The model under review builds one solid part; all positions refer to its coordinate system, in mm. A direction names the side the tool comes from. Round coordinates to 2 decimals unless told otherwise and drop trailing zeros. Order: outer loops, then holes, each group sorted by start corner. A loop starts at its lowest first (then second) coordinate and runs counter-clockwise, first axis right, second up. Notation, with made-up numbers: (43, 39.5) -> (95, 39.5) arc R7 ccw to (95, 45.5) -> close; hole circle Ø10 at (26.25, -31.5). An arc over 180 degrees is marked (long way). Use a Markdown table: item, result. Add a question column.
```python
from build123d import *

# Parameters (mm, degrees)
CROQUIS1_W              = 50
CROQUIS1_H              = 44
SALIENTE_EXTRUIR1_DEPTH = 10
CROQUIS2_W              = 58
CROQUIS2_H              = 22.5
CORTAR_EXTRUIR2_DEPTH   = 2
CROQUIS3_W              = 25
CROQUIS3_H              = 22.5
CORTAR_EXTRUIR3_DEPTH   = 4
CROQUIS4_R              = 1.1
CORTAR_EXTRUIR4_DEPTH   = 5
CROQUIS5_R              = 1.1
CORTAR_EXTRUIR5_DEPTH   = 5
REDONDEO1_R             = 2
REDONDEO2_R             = 1


with BuildPart() as part:
    # Croquis1 → Saliente-Extruir1 (new body)
    with BuildSketch(Plane(origin=(0, 0, 0), x_dir=(1, 0, 0), z_dir=(0, 1, 0))):
        Rectangle(CROQUIS1_W, CROQUIS1_H)
    extrude(amount=SALIENTE_EXTRUIR1_DEPTH)

    # Croquis2 → Cortar-Extruir2 (cut)
    with BuildSketch(Plane(origin=(0, 10, 0), x_dir=(1, 0, 0), z_dir=(0, 1, 0))):
        Rectangle(CROQUIS2_W, CROQUIS2_H)
    extrude(amount=-CORTAR_EXTRUIR2_DEPTH, mode=Mode.SUBTRACT)

    # Croquis3 → Cortar-Extruir3 (cut)
    with BuildSketch(Plane(origin=(0, 8, 0), x_dir=(1, 0, 0), z_dir=(0, 1, 0))):
        Rectangle(CROQUIS3_W, CROQUIS3_H)
    extrude(amount=-CORTAR_EXTRUIR3_DEPTH, mode=Mode.SUBTRACT)

    # Croquis4 → Cortar-Extruir4 (cut)
    with BuildSketch(Plane(origin=(0, 8, 0), x_dir=(1, 0, 0), z_dir=(0, 1, 0))):
        with Locations(Location((-22.5, 8, 0), (0, 0, 270))):
            Circle(CROQUIS4_R)
        with Locations(Location((-22.5, -8, 0), (0, 0, 270))):
            Circle(CROQUIS4_R)
        with Locations(Location((22.5, 8, 0), (0, 0, 270))):
            Circle(CROQUIS4_R)
        with Locations(Location((22.5, -8, 0), (0, 0, 270))):
            Circle(CROQUIS4_R)
    extrude(amount=-CORTAR_EXTRUIR4_DEPTH, mode=Mode.SUBTRACT)

    # Croquis5 → Cortar-Extruir5 (cut)
    with BuildSketch(Plane(origin=(0, 10, 0), x_dir=(1, 0, 0), z_dir=(0, 1, 0))):
        with Locations(Location((0, 16.625, 0), (0, 0, 270))):
            Circle(CROQUIS5_R)
        with Locations(Location((0, -16.625, 0), (0, 0, 270))):
            Circle(CROQUIS5_R)
    extrude(amount=-CORTAR_EXTRUIR5_DEPTH, mode=Mode.SUBTRACT)

    # Redondeo1
    redondeo1_edges = [part.edges().sort_by_distance(p)[0] for p in [
        (-25, 5, -22),
        (25, 5, -22),
        (25, 5, 22),
        (-25, 5, 22),
    ]]
    fillet(redondeo1_edges, radius=REDONDEO1_R)

    # Redondeo2
    redondeo2_edges = [part.edges().sort_by_distance(p)[0] for p in [
        (0, 10, 11.25),
        (0, 10, -11.25),
    ]]
    fillet(redondeo2_edges, radius=REDONDEO2_R)


solid = part.part
```
Q1. Add section B-B (z = 8). Write out the cut boundary in (x, y).
Q2. Insertion check: pin 1 (1.8 mm diameter, centred on x = 22.5, z = -7.5, fed in from +Y); pin 2 (7 mm diameter, centred on x = 4, z = -3, fed in from +Y). Each pin has a flat end and moves straight along its axis. Give the tip position at first contact, or say it passes through.
Q3. Mouldability with a two-part tool opening along X and no side actions: class faces 1 (the cylindrical face through (21.426, 5.535, 7.762)), 2 (the flat face through (0, 7, -11.25)), 3 (the flat face through (-19, 8, 0)), 4 (the cylindrical face through (24.4, 5.07, 21.43)) as pulls with the +X half, pulls with the -X half, needs draft (parallel to the pull), parting line crosses it, or undercut.
Q4. Machinability: for faces 5 (the flat face through (23, 3, 8)), 6 (the flat face through (0, 10, -18)), which of the approach directions +Z, -Z, +X, -X, +Y, -Y give a long, thin tool a straight path to every point of the face, cutting with its end or side? Answer none if there is none.
Q5. Wall thickness on line 1 (X direction, y = 5.7, z = 8); line 2 (Z direction, x = 5, y = 8.25); line 3 (Y direction, x = 9.5, z = 9): over which ranges is each line inside the solid? List them lowest first. Write a range as [from, to].
Q6. Add section D-D (x = -20). Write out the cut boundary in (y, z).
Q7. Add section A-A (y = 6). Write out the cut boundary in (x, z) (3 decimals).
Q8. Add section C-C (x = -2). Write out the cut boundary in (y, z).
Report:
| question | item | result |
|---|---|---|
| 1 | outline | (-25, 0) -> (25, 0) -> (25, 8) -> (23.6, 8) -> (23.6, 3) -> (21.4, 3) -> (21.4, 8) -> (12.5, 8) -> (12.5, 4) -> (-12.5, 4) -> (-12.5, 8) -> (-21.4, 8) -> (-21.4, 3) -> (-23.6, 3) -> (-23.6, 8) -> (-25, 8) -> close |
| 2 | pin 1 | stops at y = 8 |
| 2 | pin 2 | stops at y = 4 |
| 3 | face 1 | undercut |
| 3 | face 2 | undercut |
| 3 | face 3 | needs draft |
| 3 | face 4 | pulls with the +X half |
| 4 | face 5 | +Y |
| 4 | face 6 | +Z, -Z, +X, -X, +Y |
| 5 | line 1 | x = [-25, -23.6], [-21.4, -12.5], [12.5, 21.4], [23.6, 25] |
| 5 | line 2 | z = [-22, -11.25], [11.25, 22] |
| 5 | line 3 | y = [0, 4] |
| 6 | outline | (0, -22) -> (10, -22) -> (10, -12.25) arc R1 ccw to (9, -11.25) -> (8, -11.25) -> (8, 11.25) -> (9, 11.25) arc R1 ccw to (10, 12.25) -> (10, 22) -> (0, 22) -> close |
| 7 | outline | (-25, -20) arc R2 ccw to (-23, -22) -> (23, -22) arc R2 ccw to (25, -20) -> (25, 20) arc R2 ccw to (23, 22) -> (-23, 22) arc R2 ccw to (-25, 20) -> close; hole circle Ø2.2 at (-22.5, -8); hole circle Ø2.2 at (-22.5, 8); hole (-12.5, -11.25) -> (12.5, -11.25) -> (12.5, 11.25) -> (-12.5, 11.25) -> close; hole circle Ø2.2 at (0, -16.625); hole circle Ø2.2 at (0, 16.625); hole circle Ø2.2 at (22.5, -8); hole circle Ø2.2 at (22.5, 8) |
| 8 | outline | (0, -22) -> (10, -22) -> (10, -12.25) arc R1 ccw to (9, -11.25) -> (4, -11.25) -> (4, 11.25) -> (9, 11.25) arc R1 ccw to (10, 12.25) -> (10, 22) -> (0, 22) -> close |
